Design review of the part built by this model. Coordinates are the model's own, in mm. A direction names the side the tool comes from. Round coordinates to 2 decimals unless told otherwise and drop trailing zeros. Write each loop counter-clockwise with the first axis right and the second up, starting at its lowest first coordinate (ties: lowest second). Pieces come first, ordered by that corner, then holes.
Autodesk Fusion 360 part; units mm, degrees
sketch "Sketch2" plane through (0, 0, 0) normal (0, 0, 1) x (1, 0, 0)
  circle A0 centre (0, 0) radius 50
  circle A1 centre (0, 0) radius 67.5
  line L0 (0, 0) -> (150, 0) construction
  line L1 (0, 0) -> (-150, 0) construction
  line L2 (-150, 0) -> (-150, 5) construction
  line L3 (-150, 0) -> (-150, -5) construction
  line L4 (-174.4949, 5) -> (-189.6863, 5)
  line L5 (-174.4949, -5) -> (-189.6863, -5)
  line L6 (150, 0) -> (150, 5) construction
  line L7 (150, 0) -> (150, -5) construction
  line L8 (174.4949, 5) -> (189.6863, 5)
  line L9 (174.4949, -5) -> (189.6863, -5)
  arc A2 (-174.4949, -5) -> (-174.4949, 5) centre (-150, 0) ccw
  arc A3 (174.4949, 5) -> (174.4949, -5) centre (150, 0) ccw
  arc A4 (-129.4737, 34.3318) -> (-58.4135, 47.0411) centre (-101.25, 81.538) ccw
  arc A5 (-58.4135, -47.0411) -> (-129.4737, -34.3318) centre (-101.25, -81.538) ccw
  arc A6 (129.4737, -34.3318) -> (58.4135, -47.0411) centre (101.25, -81.538) ccw
  arc A7 (58.4135, 47.0411) -> (129.4737, 34.3318) centre (101.25, 81.538) ccw
  arc A8 (-189.6863, -5) -> (-129.4737, -34.3318) centre (-150, 0) ccw
  arc A9 (-129.4737, 34.3318) -> (-189.6863, 5) centre (-150, 0) ccw
  arc A10 (189.6863, 5) -> (129.4737, 34.3318) centre (150, 0) ccw
  arc A11 (129.4737, -34.3318) -> (189.6863, -5) centre (150, 0) ccw
  arc A12 (-58.4135, -47.0411) -> (58.4135, -47.0411) centre (0, 0) ccw
  arc A13 (58.4135, 47.0411) -> (-58.4135, 47.0411) centre (0, 0) ccw
  dimension "d13" = 100
  dimension "d14" = 135
  dimension "d15" = 150
  dimension "d16" = 150
  dimension "d17" = 150
  dimension "d18" = 50
  dimension "d19" = 80
  dimension "d20" = 50
  dimension "d21" = 80
  dimension "d22" = 5
  dimension "d23" = 5
  dimension "d24" = 5
  dimension "d25" = 5
  dimension "d26" = 110
  dimension "d27" = 110
  dimension "d28" = 110
  dimension "d30" = 110
extrude "Extrude2" add sketch "Sketch2" along normal blind 10 contours A1
extrude "Extrude3" add sketch "Sketch2" along normal blind 20 contours L4 L5 L8 L9 A2 A3 A4 A5 A6 A7 A8 A9 A10 A11 A12 A13
1) For P1, Ø7.5, axis at x = -179.5, z = 12, coming from the +Y side; P2, Ø5, axis at y = 15, z = 3.5, coming from the -X side; P3, Ø3, axis at x = -58, z = 11, coming from the -Y side, all flat-tipped, find the tip position at first contact; note any pin that passes through.
2) For line 1 along Y through (x, z) = (150, 6.75); line 2 along X through (y, z) = (-9.5, 3.5); line 3 along X through (y, z) = (10, 16.5), list the stretches that pass through material, from the lowest coordinate up.
3) Add section B-B on x = 0. State the section outline as (y, z) points.
4) Add section D-D on y = 20. State the section outline as (x, z) points.
5) The part is to be moulded in two halves that separate along Y. For faces 4 (the face through (-91, 27.5, 9.9)), 5 (the face through (-125.02, 1.03, 9.86)), 6 (the face through (168.02, -35.71, 9.86)), say which applies: pulls with the +Y half, pulls with the -Y half, needs draft (parallel to the pull), parting line crosses it, or undercut.
6) Add section C-C on z = 6.5. State the section outline as (x, y) points.
7) Add section A-A on y = 0. State the section outline as (x, z) points.
8) For faces 1 (the face through (0.937, -74.994, 9.86)), 2 (the face through (-53.57, 41.07, 14.93)), 3 (the face through (182, 5, 10)), list the 3-axis set-ups (+Z, -Z, +X, -X, +Y, -Y) from which the entire face can be reached by the end or side of a thin tool; tool diameter is ignored.
Computed:
1. P1: stops at y = 30.61
1. P2: stops at x = -188
1. P3: stops at y = -49.32
2. line 1: y = -40 to -25, 25 to 40
2. line 2: x = -188.86 to -173.12, -126.88 to -49.09, 49.09 to 126.88, 173.12 to 188.86
2. line 3: x = -188.73 to -172.91, -127.09 to -66.76, 66.76 to 127.09, 172.91 to 188.73
3. outline: (-75, 0) - (-50, 0) - (-50, 10) - (-67.5, 10) - (-67.5, 20) - (-75, 20) - close; (50, 0) - (75, 0) - (75, 20) - (67.5, 20) - (67.5, 10) - (50, 10) - close
4. outline: (-184.64, 0) - (-165, 0) - (-165, 20) - (-184.64, 20) - close; (-135, 0) - (-45.83, 0) - (-45.83, 10) - (-64.47, 10) - (-64.47, 20) - (-135, 20) - close; (45.83, 0) - (135, 0) - (135, 20) - (64.47, 20) - (64.47, 10) - (45.83, 10) - close; (165, 0) - (184.64, 0) - (184.64, 20) - (165, 20) - close
5. face 4: pulls with the +Y half
5. face 5: undercut
5. face 6: pulls with the -Y half
6. outline: (-189.69, -5) arc R40 ccw to (-129.47, -34.33) arc R55 cw to (-58.41, -47.04) arc R75 ccw to (58.41, -47.04) arc R55 cw to (129.47, -34.33) arc R40 ccw to (189.69, -5) - (174.49, -5) arc R25 cw (long way) to (174.49, 5) - (189.69, 5) arc R40 ccw to (129.47, 34.33) arc R55 cw to (58.41, 47.04) arc R75 ccw to (-58.41, 47.04) arc R55 cw to (-129.47, 34.33) arc R40 ccw to (-189.69, 5) - (-174.49, 5) arc R25 cw (long way) to (-174.49, -5) - close; hole circle Ø100 at (0, 0)
7. outline: (-125, 0) - (-50, 0) - (-50, 10) - (-67.5, 10) - (-67.5, 20) - (-125, 20) - close; (50, 0) - (125, 0) - (125, 20) - (67.5, 20) - (67.5, 10) - (50, 10) - close
8. face 1: +Z, -Z, -Y
8. face 2: +Z
8. face 3: +Z, -Z, +X
